from build123d import *

# Parameters (mm, degrees)
SKETCH_2_W      = 500
SKETCH_2_H      = 400
EXTRUDE_1_DEPTH = 200
SKETCH_3_R      = 40
EXTRUDE_2_DEPTH = 10
SKETCH_3_3_R    = 40
EXTRUDE_3_DEPTH = 20


with BuildPart() as part:
    # Sketch 2 → Extrude 1 (new body)
    with BuildSketch(Plane(origin=(0, 0, 0), x_dir=(1, 0, 0), z_dir=(0, 1, 0))):
        Rectangle(SKETCH_2_W, SKETCH_2_H)
    extrude(amount=EXTRUDE_1_DEPTH)

    # Sketch 3 → Extrude 2 (add)
    with BuildSketch(Plane(origin=(250, 0, 0), x_dir=(0, 0, -1), z_dir=(1, 0, 0))):
        with Locations(Location((80, 100, 0), (0, 0, 180))):
            Circle(SKETCH_3_R)
    extrude_2 = extrude(amount=EXTRUDE_2_DEPTH)

    # Sketch 3_3 → Extrude 3 (add)
    with BuildSketch(Plane(origin=(250, 0, 0), x_dir=(0, 0, -1), z_dir=(1, 0, 0))):
        with Locations((-80, 100)):
            Circle(SKETCH_3_3_R)
    extrude_3 = extrude(amount=EXTRUDE_3_DEPTH)

    # Mirror 1: Extrude 2, Extrude 3 across plane
    add(extrude_2.mirror(Plane(origin=(0, 0, 0), x_dir=(0, 0, 1), z_dir=(1, 0, 0))))
    add(extrude_3.mirror(Plane(origin=(0, 0, 0), x_dir=(0, 0, 1), z_dir=(1, 0, 0))))


solid = part.part
Design review of the part built by this model. Coordinates are the model's own, in mm. A direction names the side the tool comes from. Coordinates: 2 decimals unless noted, no trailing zeros. Order: outer loops, then holes, each group sorted by start corner. A loop starts at its lowest first (then second) coordinate and runs counter-clockwise, first axis right, second up. Notation, with made-up numbers: (39, 15.5) -> (48, 15.5) arc R20 cw to (48, 19.5) -> close; hole circle Ø3 at (88, 28). An arc over 180 degrees is marked (long way). One line per item, written item: value.
1) We need section B-B, the plane y = 100. Give the boundary of the cut face in (x, z).
Output values:
outline: (-270, 40) -> (-250, 40) -> (-250, -40) -> (-260, -40) -> (-260, -120) -> (-250, -120) -> (-250, -200) -> (250, -200) -> (250, -120) -> (260, -120) -> (260, -40) -> (250, -40) -> (250, 40) -> (270, 40) -> (270, 120) -> (250, 120) -> (250, 200) -> (-250, 200) -> (-250, 120) -> (-270, 120) -> close
2) To check wall thickness, follow probe 1 along X at (y, z) = (162, -102); probe 2 along X at (y, z) = (101.5, -98.5). State the ranges of each line that lie inside material, in increasing order. Write a range as [from, to].
Output values:
probe 1: x = [-250, 250]
probe 2: x = [-260, 260]
3) We need section D-D, the plane y = 20. Give the boundary of the cut face in (x, z).
Output values:
outline: (-250, -200) -> (250, -200) -> (250, 200) -> (-250, 200) -> close
4) Clearance check with flat-ended pins moving along their axes: P1, Ø5, axis at y = 179, z = -25, coming from the +X side; P2, Ø1.5, axis at y = 43, z = -53, coming from the -X side; P3, Ø24, axis at y = 93.5, z = -77.5, coming from the +X side. State where each tip first meets the part, or that it passes through.
Output values:
P1: stops at x = 250
P2: stops at x = -250
P3: stops at x = 260
5) We need section A-A, the plane z = 80. Give the boundary of the cut face in (x, y).
Output values:
outline: (-270, 60) -> (-250, 60) -> (-250, 0) -> (250, 0) -> (250, 60) -> (270, 60) -> (270, 140) -> (250, 140) -> (250, 200) -> (-250, 200) -> (-250, 140) -> (-270, 140) -> close
6) We need section C-C, the plane z = -80. Give the boundary of the cut face in (x, y).
Output values:
outline: (-260, 60) -> (-250, 60) -> (-250, 0) -> (250, 0) -> (250, 60) -> (260, 60) -> (260, 140) -> (250, 140) -> (250, 200) -> (-250, 200) -> (-250, 140) -> (-260, 140) -> close
7) Machinability: for faces 1 (the face through (260, 99, -81)), 2 (the face through (250, 99, 3)), 3 (the face through (-259.86, 112.015, 41.847)), which of the approach directions +Z, -Z, +X, -X, +Y, -Y give a long, thin tool a straight path to every point of the face, cutting with its end or side? Answer none if there is none.
Output values:
face 1: -Z, +X, +Y, -Y
face 2: +X
face 3: -X
